```python
from build123d import *

# Parameters (mm, degrees)
F0_R     = 117.5
F0_R_2   = 11
F0_R_3   = 21.5
F0_R_4   = 17.5
F1_DEPTH = 5
F2_R     = 7
F3_DEPTH = 5.001
F4_R     = 4
F5_DEPTH = 5.001


with BuildPart() as f1:
    # F0 (on Top) → F1 (new body)
    with BuildSketch(Plane.XY):
        Circle(F0_R)
        with Locations((-4.196429, -36.928568)):
            Circle(F0_R_2, mode=Mode.SUBTRACT)
        with Locations((-22, 0)):
            Circle(F0_R_3, mode=Mode.SUBTRACT)
        with Locations((-5.203568, 36.592856)):
            Circle(F0_R_2, mode=Mode.SUBTRACT)
        with Locations((27, 0)):
            Circle(F0_R_4, mode=Mode.SUBTRACT)
    extrude(amount=F1_DEPTH)

    # F2 (on face) → F3 (cut, through all)
    with BuildSketch(Plane(origin=(0, 0, 0), x_dir=(1, 0, 0), z_dir=(0, 0, -1))):
        with Locations((-100, 0)):
            Circle(F2_R)
        with Locations((0, 100)):
            Circle(F2_R)
        with Locations((100, 0)):
            Circle(F2_R)
        with Locations((0, -100)):
            Circle(F2_R)
    extrude(amount=-F3_DEPTH, mode=Mode.SUBTRACT)

    # F4 (on face) → F5 (cut, through all)
    with BuildSketch(Plane.XY.offset(5)):
        with Locations((24.09021, 34.404386)):
            Circle(F4_R)
    extrude(amount=-F5_DEPTH, mode=Mode.SUBTRACT)


solid = f1.part
```
CAD build for the part. Positions are in the model's coordinates, mm. Coordinates: 2 decimals unless noted, no trailing zeros. Write each loop counter-clockwise with the first axis right and the second up, starting at its lowest first coordinate (ties: lowest second). Pieces come first, ordered by that corner, then holes.
(1) Drill centre lines: probe 1 along Y at (x, z) = (1, 4.35); probe 2 along Y at (x, z) = (-3.5, 2.8); probe 3 along X at (y, z) = (6, 1.35). Where is each one in solid material? Low to high.
(2) Cut at A-A, the plane y = 0. List the corners of the cut face in (x, z), and give its area (3 significant figures).
(3) Flat gauge pins, fed straight in: pin 1 (16 mm diameter, centred on x = 0, y = 100, fed in from +Z); pin 2 (17.5 mm diameter, centred on x = -5.2, y = 36.59, fed in from +Z); pin 3 (2 mm diameter, centred on x = 57.5, z = 3.5, fed in from +Y); pin 4 (3 mm diameter, centred on x = 28, z = 1.5, fed in from +Y). Where does each tip first touch, or does it go through?
(4) Two-plate mould, pull along X, no slides. Class faces 1 (the face through (-2, -24, 5)), 2 (the face through (-1.493, 6.458, 2.465)), 3 (the face through (-15.3, 116.5, 2.5)): +X half, -X half, draft (parallel to the pull), parting line (faces both ways), or undercut.
(5) Cut at B-B, the plane x = -22. List the corners of the cut face in (y, z).
(6) Cut at C-C, the plane y = -33.5. List the corners of the cut face in (x, z), and give its area (3 significant figures).
(7) Cut at D-D, the plane z = 3.95. Count the separate pieces of the cut face and the enclosed holes in it, and give its area (3 significant figures).
Geometry says:
1. probe 1: y = -117.5 to -106.93, -93.07 to -46.62, -27.23 to 27.51, 45.68 to 93.07, 106.93 to 117.5
1. probe 2: y = -117.45 to -106.06, -93.94 to -47.91, -25.95 to -10.95, 10.95 to 25.73, 47.46 to 93.94, 106.06 to 117.45
1. probe 3: x = -117.35 to -103.61, -96.39 to -42.65, -1.35 to 10.56, 43.44 to 96.39, 103.61 to 117.35
2. outline: (-117.5, 0) - (-107, 0) - (-107, 5) - (-117.5, 5) - close; (-93, 0) - (-43.5, 0) - (-43.5, 5) - (-93, 5) - close; (-0.5, 0) - (9.5, 0) - (9.5, 5) - (-0.5, 5) - close; (44.5, 0) - (93, 0) - (93, 5) - (44.5, 5) - close; (107, 0) - (117.5, 0) - (117.5, 5) - (107, 5) - close
2. area: 645 mm2
3. pin 1: stops at z = 5
3. pin 2: passes through
3. pin 3: stops at y = 103.02
3. pin 4: stops at y = 114.47
4. face 1: draft
4. face 2: undercut
4. face 3: parting line
5. outline: (-115.42, 0) - (-21.5, 0) - (-21.5, 5) - (-115.42, 5) - close; (21.5, 0) - (115.42, 0) - (115.42, 5) - (21.5, 5) - close
6. outline: (-112.62, 0) - (-14.65, 0) - (-14.65, 5) - (-112.62, 5) - close; (6.26, 0) - (112.62, 0) - (112.62, 5) - (6.26, 5) - close
6. area: 1,020 mm2
7. separate pieces: 1
7. enclosed holes: 9
7. area: 39,500 mm2
